```python
from build123d import *

# Parameters (mm, degrees)
F1_DEPTH = 1244.6
F2_R     = 5.08
F3_R     = 8.89


with BuildPart() as f1:
    # F0 (on Right) → F1 (new body)
    with BuildSketch(Plane.YZ):
        Polygon((0, 76.2), (0, 0), (38.0492, 0), (38.0492, 6.9342), (6.5532, 12.7), (6.5532, 63.5), (38.0492, 69.2658), (38.0492, 76.2), align=None)
    extrude(amount=-F1_DEPTH)

    # F2
    f2_edges = [f1.edges().sort_by_distance(p)[0] for p in [
        (-622.3, 38.0492, 69.2658),
        (-622.3, 38.0492, 6.9342),
    ]]
    fillet(f2_edges, radius=F2_R)

    # F3
    f3_edges = [f1.edges().sort_by_distance(p)[0] for p in [
        (-622.3, 6.5532, 12.7),
        (-622.3, 6.5532, 63.5),
    ]]
    fillet(f3_edges, radius=F3_R)


solid = f1.part
```
Input: part model. Units: mm. Frame: model coordinates. A direction names the side the tool comes from. Coordinates: 2 decimals unless noted, no trailing zeros. Loops run counter-clockwise (first coordinate to the right, second up) from the corner with the lowest first, then second, coordinate; pieces in that order, holes last. Notation, with made-up numbers: M -28,51 L -22,51 A11 ccw -22,66 Z; hole C 4.25,-28 d3. An arc over 180 degrees is marked long. Use a Markdown table: item, result. Add a question column.
1) Set-up query: faces 1 (the flat face through (-1244.6, 6, 39)), 2 (the flat face through (-613.588, 24.003, 9.505)). Return all of +Z, -Z, +X, -X, +Y, -Y with unobstructed straight access to the full face (end or side cutting, diameter ignored); none if empty.
2) Line query: L1, parallel to Z at x = -397, y = 13; L2, parallel to Z at x = -98, y = 13.5; L3, parallel to Y at x = -1159.5, z = 35. Output: solid intervals per line, ascending. Write a range as from..to.
3) Draft query along Z for faces 3 (the flat face through (-614, 19, 76.2)), 4 (the flat face through (-614, 0, 39)), 5 (the flat face through (-614, 6.553, 38)). Return one class per face: +Z half, -Z half, draft (parallel to the pull), parting line (faces both ways), or undercut.
4) Section A-A, the plane x = -894.5. Return the cut outline in (y, z), plus the area to 3 significant figures.
5) Section B-B, the plane z = 38. Return the cut outline in (x, y).
6) Pin query (flat end, axial travel): P1, Ø11, axis at x = -779, z = 36.5, coming from the +Y side. Return the tip coordinate at first contact, or that it passes through.
Answer below:
| question | item | result |
|---|---|---|
| 1 | face 1 | +Z, -Z, -X, +Y, -Y |
| 1 | face 2 | +X, -X, +Y |
| 2 | L1 | 0..11.56, 64.64..76.2 |
| 2 | L2 | 0..11.44, 64.76..76.2 |
| 2 | L3 | 0..6.55 |
| 3 | face 3 | +Z half |
| 3 | face 4 | draft |
| 3 | face 5 | undercut |
| 4 | outline | M 0,0 L 38.05,0 L 38.05,2.7 A5.08 ccw 33.88,7.7 L 13.84,11.37 A8.89 cw 6.55,20.11 L 6.55,56.09 A8.89 cw 13.84,64.83 L 33.88,68.5 A5.08 ccw 38.05,73.5 L 38.05,76.2 L 0,76.2 Z |
| 4 | area | 1,130 mm2 |
| 5 | outline | M -1244.6,0 L 0,0 L 0,6.55 L -1244.6,6.55 Z |
| 6 | P1 | y = 6.55 |
